Check sheet for the modelled part. Datum: model origin and axes. Units: mm. A direction names the side the tool comes from. Round coordinates to 2 decimals unless told otherwise and drop trailing zeros. Write each loop counter-clockwise with the first axis right and the second up, starting at its lowest first coordinate (ties: lowest second). Pieces come first, ordered by that corner, then holes. Notation, with made-up numbers: M -28.5,-3.75 L 20.5,-3.75 A18 cw 20.5,10.25 Z; hole C -16,-5.5 d9. An arc over 180 degrees is marked long. One line per item, written item: value.
from build123d import *

# Parameters (mm, degrees)
F0_W     = 80
F0_H     = 58
F0_R     = 20
F1_DEPTH = 60
F2_R     = 4.25
F3_DEPTH = 58.001
F2_R_2   = 7
F4_DEPTH = 16


with BuildPart() as f1:
    # F0 (on Top) → F1 (new body)
    with BuildSketch(Plane.XY):
        Rectangle(F0_W, F0_H)
        Circle(F0_R, mode=Mode.SUBTRACT)
    extrude(amount=F1_DEPTH)

    # F2 (on face) → F3 (cut, through all)
    with BuildSketch(Plane(origin=(0, 29, 0), x_dir=(-1, 0, 0), z_dir=(0, 1, 0))):
        with Locations((30, 13)):
            Circle(F2_R)
        with Locations((-30, 13)):
            Circle(F2_R)
        with Locations((-30, 47)):
            Circle(F2_R)
        with Locations((30, 47)):
            Circle(F2_R)
    extrude(amount=-F3_DEPTH, mode=Mode.SUBTRACT)

    # F2 (on face) → F4 (cut)
    with BuildSketch(Plane(origin=(0, 29, 0), x_dir=(-1, 0, 0), z_dir=(0, 1, 0))):
        with Locations((30, 13)):
            Circle(F2_R_2)
        with Locations((30, 13)):
            Circle(F2_R, mode=Mode.SUBTRACT)
        with Locations((-30, 13)):
            Circle(F2_R_2)
        with Locations((-30, 13)):
            Circle(F2_R, mode=Mode.SUBTRACT)
        with Locations((-30, 47)):
            Circle(F2_R_2)
        with Locations((-30, 47)):
            Circle(F2_R, mode=Mode.SUBTRACT)
        with Locations((30, 47)):
            Circle(F2_R_2)
        with Locations((30, 47)):
            Circle(F2_R, mode=Mode.SUBTRACT)
    extrude(amount=-F4_DEPTH, mode=Mode.SUBTRACT)


solid = f1.part
Q1. Sectioned sample at B-B on y = 0. Enter the section's corners in (x, z), and give its area (3 significant figures).
Completed:
outline: M -40,0 L -20,0 L -20,60 L -40,60 Z; M 20,0 L 40,0 L 40,60 L 20,60 Z; hole C -30,13 d8.5; hole C -30,47 d8.5; hole C 30,13 d8.5; hole C 30,47 d8.5
area: 2,170 mm^2
Q2. Sectioned sample at A-A on z = 47. Enter the section's corners in (x, y), and give its area (3 significant figures).
Completed:
outline: M -40,-29 L -34.25,-29 L -34.25,13 L -37,13 L -37,29 L -40,29 Z; M -25.75,-29 L 25.75,-29 L 25.75,13 L 23,13 L 23,29 L -23,29 L -23,13 L -25.75,13 Z; M 34.25,-29 L 40,-29 L 40,29 L 37,29 L 37,13 L 34.25,13 Z; hole C 0,0 d40
area: 2,220 mm^2
Q3. Scan lines: line 1 (Z direction, x = 30, y = -10); line 2 (Z direction, x = -30, y = 22.25); line 3 (Y direction, x = 16.5, z = 4). Record each from-to range of solid material in increasing order. Write a range as [from, to].
Completed:
line 1: [0, 8.75], [17.25, 42.75], [51.25, 60]
line 2: [0, 6], [20, 40], [54, 60]
line 3: [-29, -11.3], [11.3, 29]
Q4. Depth check by flat-ended pin: P1, Ø7, axis at x = -32.5, z = 48.5, coming from the +Y side. Enter the tip coordinate at first touch or a pass-through.
Completed:
P1: y = 13
Q5. Access from +Z, -Z, +X, -X, +Y, -Y to the whole of each face (thin tool, end or side, straight path). Record for faces 1 (the cylindrical face through (-36.466, 21.112, 10.319)), 2 (the flat face through (-9, 20, 0)).
Completed:
face 1: +Y
face 2: -Z, +X, -X, +Y, -Y
Q6. Sectioned sample at C-C on x = -30. Enter the section's corners in (y, z).
Completed:
outline: M -29,0 L 29,0 L 29,6 L 13,6 L 13,8.75 L -29,8.75 Z; M -29,17.25 L 13,17.25 L 13,20 L 29,20 L 29,40 L 13,40 L 13,42.75 L -29,42.75 Z; M -29,51.25 L 13,51.25 L 13,54 L 29,54 L 29,60 L -29,60 Z
Q7. Draft check along X on faces 3 (the flat face through (-1, -29, 30)), 4 (the flat face through (40, 0, 30)), 5 (the flat face through (-40, 0, 30)), 6 (the cylindrical face through (-4.336, -19.524, 29.58)). Enter one of: pulls with the +X half, pulls with the -X half, needs draft (parallel to the pull), parting line crosses it, or undercut.
Completed:
face 3: needs draft
face 4: pulls with the +X half
face 5: pulls with the -X half
face 6: undercut
Q8. Sectioned sample at D-D on y = 25.5. Enter the section's corners in (x, z).
Completed:
outline: M -40,0 L 40,0 L 40,60 L -40,60 Z; hole C -30,13 d14; hole C -30,47 d14; hole C 30,13 d14; hole C 30,47 d14
